```python
from build123d import *

# Parameters (mm, degrees)
F1_DEPTH = 65
F2_R     = 9
F3_R     = 18
F4_SIZE  = 5


with BuildPart() as f1:
    # F0 (on Front) → F1 (new body)
    with BuildSketch(Plane.XZ):
        Polygon((0, 9), (0, 0), (165, 0), (165, 65), (156, 65), (156, 9), align=None)
    extrude(amount=-F1_DEPTH)

    # F2
    f2_edges = [f1.edges().sort_by_distance(p)[0] for p in [
        (156, 32.5, 9),
    ]]
    fillet(f2_edges, radius=F2_R)

    # F3
    f3_edges = [f1.edges().sort_by_distance(p)[0] for p in [
        (165, 32.5, 0),
    ]]
    fillet(f3_edges, radius=F3_R)

    # F4
    f4_edges = [f1.edges().sort_by_distance(p)[0] for p in [
        (160.5, 65, 65),
        (160.5, 0, 65),
        (0, 65, 4.5),
        (0, 0, 4.5),
    ]]
    chamfer(f4_edges, length=F4_SIZE)


solid = f1.part
```
For this review, take the finished solid that the model builds, in its own axes (mm). A direction names the side the tool comes from. Coordinates: 2 decimals unless noted, no trailing zeros. Write each loop counter-clockwise with the first axis right and the second up, starting at its lowest first coordinate (ties: lowest second). Pieces come first, ordered by that corner, then holes. Notation, with made-up numbers: (44.5, 60.5) - (103.5, 60.5) arc R32 cw to (103.5, 95.5) - close; hole circle Ø3 at (33.5, -5.75). An arc over 180 degrees is marked (long way). Answer in a Markdown table with one row per item. Add a question column.
Q1. For P1, Ø3, axis at y = 44.5, z = 37.5, coming from the -X side; P2, Ø5, axis at x = 66, y = 11.5, coming from the +Z side, all flat-tipped, find the tip position at first contact; note any pin that passes through.
Q2. For probe 1 along X at (y, z) = (46, 54.5); probe 2 along Z at (x, y) = (84.5, 16); probe 3 along X at (y, z) = (3.5, 11), list the stretches that pass through material, from the lowest coordinate up.
Q3. We need section A-A, the plane y = 23.5. State the section outline as (x, z) points.
Q4. Tool access review of faces 1 (the flat face through (72, 32, 0)), 2 (the flat face through (156, 32, 42)): name each direction out of +Z, -Z, +X, -X, +Y, -Y from which nothing blocks a thin tool from reaching the whole face with its end or side.
Q5. We need section C-C, the plane z = 44. State the section outline as (x, y) points, and give its area (3 significant figures).
Q6. We need section B-B, the plane x = 128.5. State the section outline as (y, z) points, and give its area (3 significant figures).
Answer list:
| question | item | result |
|---|---|---|
| 1 | P1 | stops at x = 156 |
| 1 | P2 | stops at z = 9 |
| 2 | probe 1 | x = 156 to 165 |
| 2 | probe 2 | z = 0 to 9 |
| 2 | probe 3 | x = 152.66 to 163.58 |
| 3 | outline | (0, 0) - (147, 0) arc R18 ccw to (165, 18) - (165, 65) - (156, 65) - (156, 18) arc R9 cw to (147, 9) - (0, 9) - close |
| 4 | face 1 | -Z, +X, -X, +Y, -Y |
| 4 | face 2 | +Z, -X, +Y, -Y |
| 5 | outline | (156, 0) - (165, 0) - (165, 65) - (156, 65) - close |
| 5 | area | 585 mm2 |
| 6 | outline | (0, 0) - (65, 0) - (65, 9) - (0, 9) - close |
| 6 | area | 585 mm2 |
